Check sheet for the modelled part. Datum: model origin and axes. Units: mm. A direction names the side the tool comes from. Round coordinates to 2 decimals unless told otherwise and drop trailing zeros. Order: outer loops, then holes, each group sorted by start corner. A loop starts at its lowest first (then second) coordinate and runs counter-clockwise, first axis right, second up. Notation, with made-up numbers: (38, 7) -> (68, 7) arc R32 cw to (68, 42) -> close; hole circle Ø6 at (-6.5, 44). An arc over 180 degrees is marked (long way). Answer in a Markdown table with one row per item.
Autodesk Inventor part; units mm, degrees
ref_plane "YZ Plane" through (0, 0, 0) normal (1, 0, 0) x (0, 1, 0)
ref_plane "XZ Plane" through (0, 0, 0) normal (0, 1, 0) x (-1, 0, 0)
ref_plane "XY Plane" through (0, 0, 0) normal (0, 0, 1) x (1, 0, 0)
sketch "Sketch1" plane through (0, 0, 0) normal (0, 1, 0) x (-1, 0, 0)
  line L0 (0, 0) -> (10, 0)
  line L1 (10, 0) -> (10, -27)
  line L2 (10, -27) -> (0, -27)
  line L3 (0, -27) -> (0, 0)
  dimension "d0" = 10
  dimension "d1" = 27
extrude "Extrusion1" add sketch "Sketch1" along normal blind 10
sketch "Sketch2" plane through (0, 10, 0) normal (0, 1, 0) x (1, 0, 0)
  line L0 (-10, 27) -> (-10, 0)
  line L1 (-10, 0) -> (-10, 5)
  circle A0 centre (-5, 5) radius 3
  point P0 (0, 0)
  dimension "d4" = 5
  dimension "d5" = 6
extrude "Extrusion2" cut sketch "Sketch2" against normal blind 10
sketch "Sketch3" plane through (0, 0, -27) normal (0, 0, -1) x (-1, 0, 0)
  line L0 (0, 10) -> (10, 10)
  line L1 (0, 10) -> (5, 10)
  line L2 (5, 10) -> (5, 5)
  circle A0 centre (5, 5) radius 1.95
  point P0 (0, 0)
  dimension "d8" = 5
  dimension "d9" = 5
  dimension "d10" = 3.9
extrude "Extrusion3" cut sketch "Sketch3" against normal blind 15
properties part number "Raket_Arme"
(1) Draft check along X on faces 1 (the flat face through (0, 5, -14)), 2 (the flat face through (-10, 5, -13)), 3 (the flat face through (-5, 5, -12)). Enter one of: pulls with the +X half, pulls with the -X half, needs draft (parallel to the pull), parting line crosses it, or undercut.
Solutions:
| item | result |
|---|---|
| face 1 | pulls with the +X half |
| face 2 | pulls with the -X half |
| face 3 | undercut |
(2) Section check C-C on y = 5. Record the boundary of the cut face in (x, z).
Solutions:
| item | result |
|---|---|
| outline | (-10, -27) -> (-6.95, -27) -> (-6.95, -12) -> (-3.05, -12) -> (-3.05, -27) -> (0, -27) -> (0, 0) -> (-10, 0) -> close; hole circle Ø6 at (-5, -5) |
(3) Tool access check on faces 4 (the flat face through (-5, 0, -13)), 5 (the cylindrical face through (-3.052, 5.086, -19.605)). Record the directions out of +Z, -Z, +X, -X, +Y, -Y that give a thin tool (end or side, any length) a straight path to the whole face; none if there is none.
Solutions:
| item | result |
|---|---|
| face 4 | +Z, -Z, +X, -X, -Y |
| face 5 | -Z |
(4) Scan lines: probe 1 along Z at (x, y) = (-5, 2.5); probe 2 along X at (y, z) = (5, -17.5); probe 3 along Y at (x, z) = (-5, -20.5). Record each from-to range of solid material in increasing order. Write a range as from..to.
Solutions:
| item | result |
|---|---|
| probe 1 | -27..-8, -2..0 |
| probe 2 | -10..-6.95, -3.05..0 |
| probe 3 | 0..3.05, 6.95..10 |
(5) Section check A-A on z = -5. Record the boundary of the cut face in (x, y).
Solutions:
| item | result |
|---|---|
| outline | (-10, 0) -> (-8, 0) -> (-8, 10) -> (-10, 10) -> close; (-2, 0) -> (0, 0) -> (0, 10) -> (-2, 10) -> close |
(6) Depth check by flat-ended pin: pin 1 Ø6 at (x, z) = (-7.5, -11) entering from -Y; pin 2 Ø1.2 at (x, y) = (-4.5, 4.5) entering from -Z. Enter the tip coordinate at first touch or a pass-through.
Solutions:
| item | result |
|---|---|
| pin 1 | y = 0 |
| pin 2 | z = -12 |
(7) Section check B-B on x = -5. Record the boundary of the cut face in (y, z).
Solutions:
| item | result |
|---|---|
| outline | (0, -27) -> (3.05, -27) -> (3.05, -12) -> (6.95, -12) -> (6.95, -27) -> (10, -27) -> (10, -8) -> (0, -8) -> close; (0, -2) -> (10, -2) -> (10, 0) -> (0, 0) -> close |
(8) Section check D-D on z = -18.5. Record the boundary of the cut face in (x, y).
Solutions:
| item | result |
|---|---|
| outline | (-10, 0) -> (0, 0) -> (0, 10) -> (-10, 10) -> close; hole circle Ø3.9 at (-5, 5) |
